Could you check a few things on this model? Use its own coordinates, in mm. A direction names the side the tool comes from. Coordinates: 2 decimals unless noted, no trailing zeros. Write each loop counter-clockwise with the first axis right and the second up, starting at its lowest first coordinate (ties: lowest second). Pieces come first, ordered by that corner, then holes.
```python
from build123d import *

# Parameters (mm, degrees)
SKETCH1_R             = 15
SKETCH1_R_2           = 11.1125
BOSS_EXTRUDE1_DEPTH   = 3.175
F_6_CLEARANCE_HOLE1_D = 3.7973
F_6_32_TAPPED_HOLE1_D = 2.7051
FILLET1_R             = 10


with BuildPart() as part:
    # Sketch1 → Boss-Extrude1 (new body)
    with BuildSketch(Plane(origin=(0, 0, 0), x_dir=(0, 0, -1), z_dir=(1, 0, 0))):
        with BuildLine():
            ThreePointArc((-91.459503782, 7.5), (-130, 0), (-91.459503782, -7.5))
            Line((-91.459503782, -7.5), (-14.260527909, -7.5))
            ThreePointArc((-14.260527909, -7.5), (0, -16.1125), (14.260527909, -7.5))
            Line((14.260527909, -7.5), (100, -7.5))
            ThreePointArc((100, -7.5), (107.5, 0), (100, 7.5))
            Line((100, 7.5), (14.260527909, 7.5))
            ThreePointArc((14.260527909, 7.5), (0, 16.1125), (-14.260527909, 7.5))
            Line((-14.260527909, 7.5), (-91.459503782, 7.5))
        make_face()
        with Locations((-110, 0)):
            Circle(SKETCH1_R, mode=Mode.SUBTRACT)
        Circle(SKETCH1_R_2, mode=Mode.SUBTRACT)
    extrude(amount=BOSS_EXTRUDE1_DEPTH)

    # #6 Clearance Hole1 (through all)
    with Locations(Plane(origin=(3.175, 0, 0), x_dir=(0, 0, -1), z_dir=(1, 0, 0))):
        with Locations((-55, 0)):
            Hole(F_6_CLEARANCE_HOLE1_D / 2)

    # #6-32 Tapped Hole1 (through all)
    with Locations(Plane(origin=(3.175, 0, 0), x_dir=(0, 0, -1), z_dir=(1, 0, 0))):
        with Locations((100, 0)):
            Hole(F_6_32_TAPPED_HOLE1_D / 2)

    # Fillet1
    fillet1_edges = [part.edges().sort_by_distance(p)[0] for p in [
        (1.5875, 7.5, 91.459503782),
        (1.5875, 7.5, 14.260527909),
        (1.5875, 7.5, -14.260527909),
        (1.5875, -7.5, -14.260527909),
        (1.5875, -7.5, 14.260527909),
        (1.5875, -7.5, 91.459503782),
    ]]
    fillet(fillet1_edges, radius=FILLET1_R)


solid = part.part
```
1. On a 3-axis mill with a long thin cutter (end or side, diameter ignored), from which of +Z, -Z, +X, -X, +Y, -Y can I reach the whole of each face in a straight line? I mean faces 1 (the face through (1.57, -0.16, -107.5)), 2 (the face through (1.61, -8.633, 90.256)), 3 (the face through (1.61, 8.633, 90.256)). Say none if no direction works.
Verdict:
face 1: -Z, +X, -X
face 2: +X, -X, -Y
face 3: +X, -X, +Y
2. I want a section at B-B on x = 1.4. Please give me the cut outline in (y, z) (1 decimal).
Verdict:
outline: (-11.7, 93.8) arc R10 cw to (-7.5, 85.6) - (-7.5, 19.4) arc R10 cw to (-10.8, 12) arc R16.1 ccw to (-10.8, -12) arc R10 cw to (-7.5, -19.4) - (-7.5, -100) arc R7.5 ccw to (7.5, -100) - (7.5, -19.4) arc R10 cw to (10.8, -12) arc R16.1 ccw to (10.8, 12) arc R10 cw to (7.5, 19.4) - (7.5, 85.6) arc R10 cw to (11.7, 93.8) arc R20 ccw (long way) to start; hole circle Ø30 at (0, 110); hole circle Ø22.2 at (0, 0); hole circle Ø3.8 at (0, 55); hole circle Ø2.7 at (0, -100)
3. I want a section at C-C on z = -35. Please give me the cut outline in (x, y) (3 decimals).
Verdict:
outline: (0, -7.5) - (3.175, -7.5) - (3.175, 7.5) - (0, 7.5) - close
4. If we mould it in two halves opening along Y, with no side actions, what happens to faces 4 (the face through (0, 0, 13)), 5 (the face through (1.57, 16.11, -0.19)), 6 (the face through (1.565, 4.506, 95.693))? For each: pulls with the +Y half, pulls with the -Y half, needs draft (parallel to the pull), parting line crosses it, or undercut.
Verdict:
face 4: needs draft
face 5: pulls with the +Y half
face 6: undercut
5. For pin 1 (1.6 mm diameter, centred on x = 1.5, z = -60.5, fed in from -Y); pin 2 (1 mm diameter, centred on y = -8, z = -4.5, fed in from +X); pin 3 (1.6 mm diameter, centred on x = 2.5, z = -71.5, fed in from +Y), each with a flat end and sliding along its axis, tell me the tip position at first contact or that it passes through.
Verdict:
pin 1: stops at y = -7.5
pin 2: passes through
pin 3: stops at y = 7.5
6. I want a section at A-A on z = 110. Please give me the cut outline in (x, y) (3 decimals).
Verdict:
outline: (0, -20) - (3.175, -20) - (3.175, -15) - (0, -15) - close; (0, 15) - (3.175, 15) - (3.175, 20) - (0, 20) - close
7. Please list where these lines run through material, in increasing order: line 1 along Y through (x, z) = (2.35, 110); line 2 along Y through (x, z) = (0.8, -1); line 3 along Z through (x, y) = (2.5, -10).
Verdict:
line 1: y = -20 to -15, 15 to 20
line 2: y = -16.08 to -11.07, 11.07 to 16.08
line 3: z = -12.77 to -4.85, 4.85 to 12.77, 92.25 to 98.82, 121.18 to 127.32
